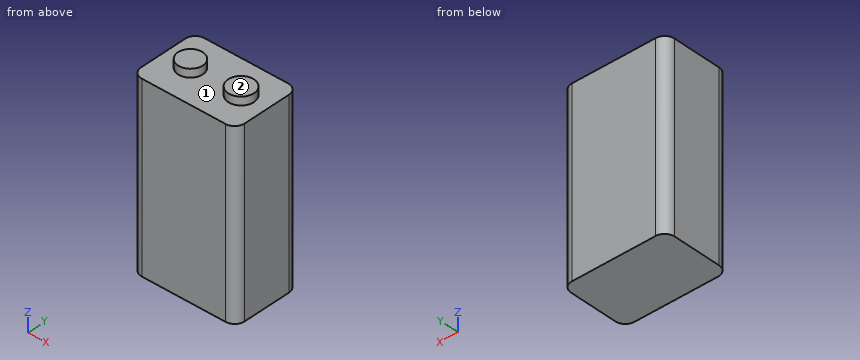
from build123d import *

# Parameters (mm, degrees)
F0_W     = 26.4922
F0_H     = 17.5006
F1_DEPTH = 46.4058
F2_R     = 3.159655
F2_R_2   = 3.294016
F3_DEPTH = 2.0828
F4_R     = 2.54


with BuildPart() as f1:
    # F0 (on Top) → F1 (new body)
    with BuildSketch(Plane.XY):
        Rectangle(F0_W, F0_H)
    extrude(amount=F1_DEPTH)

    # F2 (on face) → F3 (join)
    with BuildSketch(Plane.XY.offset(46.4058)):
        with Locations((-6.283553, 0)):
            Circle(F2_R)
        with Locations((6.670447, 0)):
            Circle(F2_R_2)
    extrude(amount=F3_DEPTH)

    # F4
    f4_edges = [f1.edges().sort_by_distance(p)[0] for p in [
        (-13.2461, -8.7503, 23.2029),
        (13.2461, -8.7503, 23.2029),
        (13.2461, 8.7503, 23.2029),
        (-13.2461, 8.7503, 23.2029),
    ]]
    fillet(f4_edges, radius=F4_R)


solid = f1.part
Can you work these out from the model? Positions are in its coordinate system, mm. Face numbers are marked on the shaded views. A direction names the side the tool comes from. Coordinates: 2 decimals unless noted, no trailing zeros. Order: outer loops, then holes, each group sorted by start corner. A loop starts at its lowest first (then second) coordinate and runs counter-clockwise, first axis right, second up. Notation, with made-up numbers: (-18.5, 80) -> (15.5, 80) arc R26 ccw to (15.5, 102) -> close; hole circle Ø8 at (-0.75, -40). An arc over 180 degrees is marked (long way). Use one line per item in the form item = value.
Q1. Which directions (+Z, -Z, +X, -X, +Y, -Y) give clear straight access to the entire face, cutting with the end or side of a thin tool? Please do the marked faces 1 and 2.
From the geometry:
face_1 = +Z
face_2 = +Z, +X, -X, +Y, -Y
Q2. Imagine slicing it at D-D, the plane y = 5. List the corners of the cut face in (x, z) for me, then the cut area to 3 significant figures.
From the geometry:
outline = (-13.25, 0) -> (13.25, 0) -> (13.25, 46.41) -> (-13.25, 46.41) -> close
area = 1,230 mm²
Q3. I need wall thicknesses on L1, parallel to Z at x = 2.25, y = 6.75; L2, parallel to X at y = -7.25, z = 36.5; L3, parallel to Y at x = -12, z = 30.5. Which ranges of each line are inside material? Lowest first, please.
From the geometry:
L1 = 0 to 46.41
L2 = -13.02 to 13.02
L3 = -8.4 to 8.4
Q4. Imagine slicing it at A-A, the plane y = 0. List the corners of the cut face in (x, z) for me.
From the geometry:
outline = (-13.25, 0) -> (13.25, 0) -> (13.25, 46.41) -> (9.96, 46.41) -> (9.96, 48.49) -> (3.38, 48.49) -> (3.38, 46.41) -> (-3.12, 46.41) -> (-3.12, 48.49) -> (-9.44, 48.49) -> (-9.44, 46.41) -> (-13.25, 46.41) -> close
Q5. Will this pin go through, and if not, where does the flat tip stop? P1, Ø3, axis at x = -0.5, y = -6.5, coming from the +Z side.
From the geometry:
P1 = 46.41
Q6. Imagine slicing it at C-C, the plane x = 4. List the corners of the cut face in (y, z) for me, then the cut area to 3 significant figures.
From the geometry:
outline = (-8.75, 0) -> (8.75, 0) -> (8.75, 46.41) -> (1.93, 46.41) -> (1.93, 48.49) -> (-1.93, 48.49) -> (-1.93, 46.41) -> (-8.75, 46.41) -> close
area = 820 mm²
Q7. Imagine slicing it at B-B, the plane x = -5.25. List the corners of the cut face in (y, z) for me.
From the geometry:
outline = (-8.75, 0) -> (8.75, 0) -> (8.75, 46.41) -> (2.99, 46.41) -> (2.99, 48.49) -> (-2.99, 48.49) -> (-2.99, 46.41) -> (-8.75, 46.41) -> close
